Design review of the part built by this model. Coordinates are the model's own, in mm. Round coordinates to 2 decimals unless told otherwise and drop trailing zeros. Loops run counter-clockwise (first coordinate to the right, second up) from the corner with the lowest first, then second, coordinate; pieces in that order, holes last. Notation, with made-up numbers: (58.25, 51) - (93.25, 51) arc R27 cw to (93.25, 85) - close; hole circle Ø11 at (49, 79). An arc over 180 degrees is marked (long way). Return JSON: item names as keys, results as strings. Group by question number.
(1) We need section C-C, the plane y = 1. Write out the cut boundary in (x, z), and give its area (3 significant figures).
(2) We need section D-D, the plane y = 56. Write out the cut boundary in (x, z).
(3) We need section B-B, the plane z = 0.3. Write out the cut boundary in (x, y).
(4) We need section A-A, the plane x = 0. Write out the cut boundary in (y, z).
(5) Wall thickness on L1, parallel to Y at x = 0, z = 0.35; L2, parallel to Y at x = -1, z = 0.1: over which ranges is each line inside the solid? List them lowest first. Write a range as [from, to].
(6) Clearance check with a flat-ended pin moving along its axis: pin 1 (5 mm diameter, centred on x = 0, y = 0, fed in from -Z). State where the tip first meets the part, or that it passes through.
from build123d import *

# Parameters (mm, degrees)
F0_R     = 2.75
F1_DEPTH = 0.4


with BuildPart() as f1:
    # F0 (on Top) → F1 (new body)
    with BuildSketch(Plane.XY):
        with BuildLine():
            Line((-5, 30), (-5, 0))
            ThreePointArc((-5, 0), (0, -5), (5, 0))
            Line((5, 0), (5, 30))
            Line((5, 30), (3.695135, 62.647687))
            ThreePointArc((3.695135, 62.647687), (0.043949, 66.197824), (-3.690581, 62.735468))
            Line((-3.690581, 62.735468), (-3.697598, 62.560059))
            Line((-3.697598, 62.560059), (-5, 30))
        make_face()
        Circle(F0_R, mode=Mode.SUBTRACT)
    extrude(amount=F1_DEPTH)


solid = f1.part
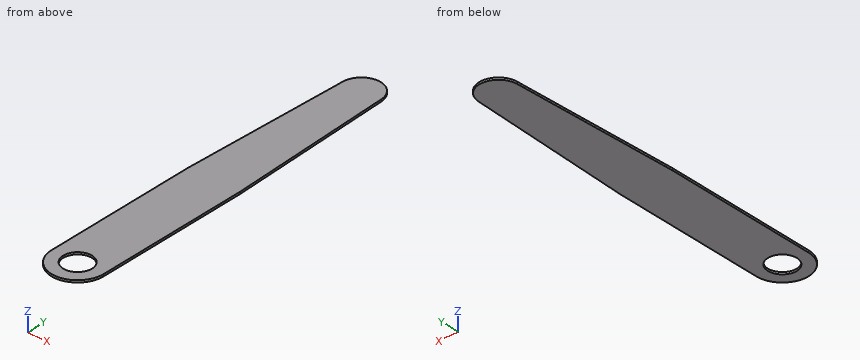
Solutions:
{
 "1": {"outline": "(-5, 0) - (-2.56, 0) - (-2.56, 0.4) - (-5, 0.4) - close; (2.56, 0) - (5, 0) - (5, 0.4) - (2.56, 0.4) - close", "area": "1.95 mm^2"},
 "2": {"outline": "(-3.96, 0) - (3.96, 0) - (3.96, 0.4) - (-3.96, 0.4) - close"},
 "3": {"outline": "(-5, 0) arc R5 ccw to (5, 0) - (5, 30) - (3.7, 62.65) arc R3.7 ccw to (-3.69, 62.74) - (-3.7, 62.56) - (-5, 30) - close; hole circle Ø5.5 at (0, 0)"},
 "4": {"outline": "(-5, 0) - (-2.75, 0) - (-2.75, 0.4) - (-5, 0.4) - close; (2.75, 0) - (66.2, 0) - (66.2, 0.4) - (2.75, 0.4) - close"},
 "5": {"L1": "[-5, -2.75], [2.75, 66.2]", "L2": "[-4.9, -2.56], [2.56, 66.06]"},
 "6": {"pin 1": "through"}
}
